Autodesk Inventor part; units mm, degrees
ref_plane "YZ Plane" through (0, 0, 0) normal (1, 0, 0) x (0, 1, 0)
ref_plane "XZ Plane" through (0, 0, 0) normal (0, 1, 0) x (-1, 0, 0)
ref_plane "XY Plane" through (0, 0, 0) normal (0, 0, 1) x (1, 0, 0)
sketch "Szkic1" plane through (0, 0, 0) normal (0, 1, 0) x (-1, 0, 0)
  line L0 (-15, -35.5) -> (15, -35.5)
  line L1 (15, -35.5) -> (15, 35.5)
  line L2 (15, 35.5) -> (-15, 35.5)
  line L3 (-15, 35.5) -> (-15, -35.5)
  line L4 (-15, -35.5) -> (15, 35.5) construction
  line L5 (15, -35.5) -> (-15, 35.5) construction
  point P0 (0, 0)
  dimension "d0" = 30
  dimension "d1" = 71
extrude "Wyciągnięcie proste1" add sketch "Szkic1" along normal blind 2
sketch "Szkic2" plane through (0, 0, 0) normal (0, -1, 0) x (1, 0, 0)
  circle A0 centre (11, 0) radius 1.5
  circle A1 centre (19, -31.5) radius 1.5
  circle A2 centre (-11, 31.5) radius 1.5
  circle A3 centre (-11, -31.5) radius 1.5
  circle A4 centre (19, 31.5) radius 1.5
  circle A5 centre (-11, 0) radius 1.5
  line L0 (23.5, -35.5) -> (-15.5, -35.5)
  line L1 (23.5, 35.5) -> (23.5, -35.5)
  line L2 (-15.5, 35.5) -> (23.5, 35.5)
  line L3 (-15.5, -35.5) -> (-15.5, 35.5)
  point P0 (0, 0)
hole "Otwór1" at (11, 0, 0) at (-11, 0, 0) at (-11, 0, 31.5) at (-11, 0, -31.5) direction (0, 1, 0) diameter 3.5 end through all
properties part number "docisk do mostka"
Part model, mm, in its own coordinate system. Coordinates: 2 decimals unless noted, no trailing zeros. Loops run counter-clockwise (first coordinate to the right, second up) from the corner with the lowest first, then second, coordinate; pieces in that order, holes last. Notation, with made-up numbers: (22.25, 56) -> (43.25, 56) arc R13 ccw to (43.25, 67) -> close; hole circle Ø3 at (-28.75, 81.5). An arc over 180 degrees is marked (long way). Use a Markdown table: item, result. Add a question column.
Item 1: Probe probe 1 along X at (y, z) = (1.3, 0); probe 2 along Z at (x, y) = (-11, 1.55); probe 3 along Z at (x, y) = (11, 1.5). List the from-to ranges inside material, lowest first.
Item 2: Band-saw the part on C-C on x = -11. Write the cut outline in (y, z), plus the area to 3 significant figures.
Item 3: Band-saw the part on A-A on z = -31.5. Write the cut outline in (x, y).
Item 4: Band-saw the part on B-B on z = 0. Write the cut outline in (x, y).
Item 5: Band-saw the part on D-D on y = 0.4. Write the cut outline in (x, z), plus the area to 3 significant figures.
Geometry says:
| question | item | result |
|---|---|---|
| 1 | probe 1 | -15 to -12.75, -9.25 to 9.25, 12.75 to 15 |
| 1 | probe 2 | -35.5 to -33.25, -29.75 to -1.75, 1.75 to 29.75, 33.25 to 35.5 |
| 1 | probe 3 | -35.5 to -1.75, 1.75 to 35.5 |
| 2 | outline | (0, -35.5) -> (2, -35.5) -> (2, -33.25) -> (0, -33.25) -> close; (0, -29.75) -> (2, -29.75) -> (2, -1.75) -> (0, -1.75) -> close; (0, 1.75) -> (2, 1.75) -> (2, 29.75) -> (0, 29.75) -> close; (0, 33.25) -> (2, 33.25) -> (2, 35.5) -> (0, 35.5) -> close |
| 2 | area | 121 mm² |
| 3 | outline | (-15, 0) -> (-12.75, 0) -> (-12.75, 2) -> (-15, 2) -> close; (-9.25, 0) -> (15, 0) -> (15, 2) -> (-9.25, 2) -> close |
| 4 | outline | (-15, 0) -> (-12.75, 0) -> (-12.75, 2) -> (-15, 2) -> close; (-9.25, 0) -> (9.25, 0) -> (9.25, 2) -> (-9.25, 2) -> close; (12.75, 0) -> (15, 0) -> (15, 2) -> (12.75, 2) -> close |
| 5 | outline | (-15, -35.5) -> (15, -35.5) -> (15, 35.5) -> (-15, 35.5) -> close; hole circle Ø3.5 at (-11, -31.5); hole circle Ø3.5 at (-11, 0); hole circle Ø3.5 at (-11, 31.5); hole circle Ø3.5 at (11, 0) |
| 5 | area | 2,090 mm² |
